from build123d import *

# Parameters (mm, degrees)
SKETCH_1_W          = 140
SKETCH_1_H          = 40
SKETCH_1_W_2        = 7
SKETCH_1_H_2        = 20
SKETCH_1_W_3        = 30
SKETCH_1_H_3        = 3.2
EXTRUDE_1_DEPTH     = 2
CUT_EXTRUDE_1_DEPTH = 3
SKETCH_3_R          = 1.55
CUT_EXTRUDE_2_DEPTH = 3


with BuildPart() as part:
    # 草图1 → 凸台-拉伸1 (new body)
    with BuildSketch(Plane(origin=(0, 0, 0), x_dir=(0, 0, -1), z_dir=(1, 0, 0))):
        Rectangle(SKETCH_1_W, SKETCH_1_H)
        with Locations((-73.5, 5)):
            Rectangle(SKETCH_1_W_2, SKETCH_1_H_2)
        with BuildLine():
            Line((-67.5, 23.2), (-35, 23.2))
            Line((-35, 23.2), (-5, 23.2))
            Line((-5, 23.2), (-5, 29.2))
            Line((-5, 29.2), (-67.5, 29.2))
            ThreePointArc((-67.5, 29.2), (-69.267766953, 28.467766953), (-70, 26.7))
            Line((-70, 26.7), (-70, 25.7))
            ThreePointArc((-70, 25.7), (-69.267766953, 23.932233047), (-67.5, 23.2))
        make_face()
        with Locations((-20, 21.6)):
            Rectangle(SKETCH_1_W_3, SKETCH_1_H_3)
        with Locations((73.5, 5)):
            Rectangle(SKETCH_1_W_2, SKETCH_1_H_2)
    extrude(amount=EXTRUDE_1_DEPTH)

    # 草图2 → 切除-拉伸1 (cut)
    with BuildSketch(Plane(origin=(2, 0, 0), x_dir=(0, 0, -1), z_dir=(1, 0, 0))):
        with BuildLine():
            Line((-65, -10), (-65, 10))
            ThreePointArc((-65, 10), (-60, 15), (-55, 10))
            Line((-55, 10), (-55, -10))
            ThreePointArc((-55, -10), (-60, -15), (-65, -10))
        make_face()
        with BuildLine():
            Line((-50, -10), (-50, 10))
            ThreePointArc((-50, 10), (-45, 15), (-40, 10))
            Line((-40, 10), (-40, -10))
            ThreePointArc((-40, -10), (-45, -15), (-50, -10))
        make_face()
        with BuildLine():
            Line((-35, -10), (-35, 10))
            ThreePointArc((-35, 10), (-30, 15), (-25, 10))
            Line((-25, 10), (-25, -10))
            ThreePointArc((-25, -10), (-30, -15), (-35, -10))
        make_face()
        with BuildLine():
            Line((-20, -10), (-20, 10))
            ThreePointArc((-20, 10), (-15, 15), (-10, 10))
            Line((-10, 10), (-10, -10))
            ThreePointArc((-10, -10), (-15, -15), (-20, -10))
        make_face()
        with BuildLine():
            Line((-5, -10), (-5, 10))
            ThreePointArc((-5, 10), (0, 15), (5, 10))
            Line((5, 10), (5, -10))
            ThreePointArc((5, -10), (0, -15), (-5, -10))
        make_face()
        with BuildLine():
            Line((10, -10), (10, 10))
            ThreePointArc((10, 10), (15, 15), (20, 10))
            Line((20, 10), (20, -10))
            ThreePointArc((20, -10), (15, -15), (10, -10))
        make_face()
        with BuildLine():
            Line((25, -10), (25, 10))
            ThreePointArc((25, 10), (30, 15), (35, 10))
            Line((35, 10), (35, -10))
            ThreePointArc((35, -10), (30, -15), (25, -10))
        make_face()
        with BuildLine():
            Line((40, -10), (40, 10))
            ThreePointArc((40, 10), (45, 15), (50, 10))
            Line((50, 10), (50, -10))
            ThreePointArc((50, -10), (45, -15), (40, -10))
        make_face()
        with BuildLine():
            Line((55, -10), (55, 10))
            ThreePointArc((55, 10), (60, 15), (65, 10))
            Line((65, 10), (65, -10))
            ThreePointArc((65, -10), (60, -15), (55, -10))
        make_face()
    extrude(amount=-CUT_EXTRUDE_1_DEPTH, mode=Mode.SUBTRACT)

    # 草图3 → 切除-拉伸2 (cut)
    with BuildSketch(Plane(origin=(2, 0, 0), x_dir=(0, 0, -1), z_dir=(1, 0, 0))):
        with Locations((-74.25, 5)):
            Circle(SKETCH_3_R)
        with Locations((74.25, 5)):
            Circle(SKETCH_3_R)
    extrude(amount=-CUT_EXTRUDE_2_DEPTH, mode=Mode.SUBTRACT)


solid = part.part
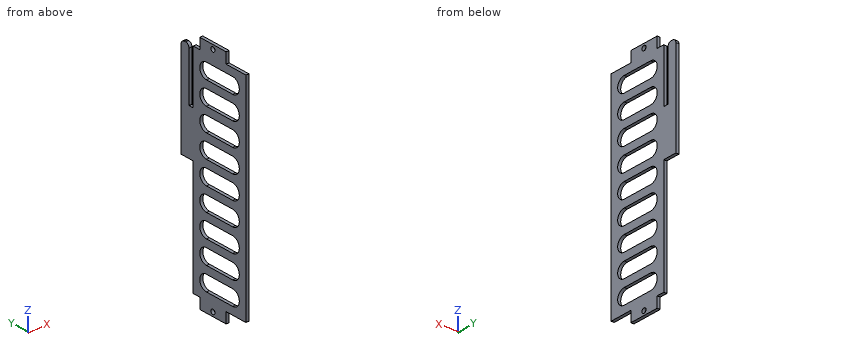
Verification items for the finished model (mm, model axes). Round coordinates to 2 decimals unless told otherwise and drop trailing zeros. Write each loop counter-clockwise with the first axis right and the second up, starting at its lowest first coordinate (ties: lowest second). Pieces come first, ordered by that corner, then holes.
(1) Material ranges on line 1 (Y direction, x = 1.2, z = -74.25); line 2 (Y direction, x = 1.85, z = 15); line 3 (Z direction, x = 1.95, y = -17.5), recorded low to high.
Returned:
line 1: y = -5 to 3.45, 6.55 to 15
line 2: y = -20 to -15, 15 to 29.2
line 3: z = -70 to 70
(2) Section check B-B (z = 45). Enter the section's corners in (x, y).
Returned:
outline: (0, -20) - (2, -20) - (2, -15) - (0, -15) - close; (0, 15) - (2, 15) - (2, 20) - (0, 20) - close; (0, 23.2) - (2, 23.2) - (2, 29.2) - (0, 29.2) - close
(3) Depth check by flat-ended pin: pin 1 Ø0.6 at (x, y) = (1, 17) entering from -Z; pin 2 Ø1 at (x, z) = (1.5, 74) entering from -Y; pin 3 Ø1 at (x, z) = (1, -29.5) entering from +Y. Enter the tip coordinate at first touch or a pass-through.
Returned:
pin 1: stops at z = -70
pin 2: stops at y = -5
pin 3: stops at y = 20
(4) Section check A-A (z = 0). Enter the section's corners in (x, y), plus the area to 3 significant figures.
Returned:
outline: (0, -20) - (2, -20) - (2, -15) - (0, -15) - close; (0, 15) - (2, 15) - (2, 20) - (0, 20) - close
area: 20.0 mm2
(5) Section check D-D (y = 18.5). Enter the section's corners in (x, z), plus the area to 3 significant figures.
Returned:
outline: (0, -70) - (2, -70) - (2, 70) - (0, 70) - close
area: 280 mm2
(6) Section check C-C (y = 0). Give the number of separate pieces and of enclosed holes in the cut face, plus the area to 3 significant figures.
Returned:
separate pieces: 10
enclosed holes: 0
area: 128 mm2
